Check sheet for the modelled part. Datum: model origin and axes. Units: mm. A direction names the side the tool comes from. Coordinates: 2 decimals unless noted, no trailing zeros. Write each loop counter-clockwise with the first axis right and the second up, starting at its lowest first coordinate (ties: lowest second). Pieces come first, ordered by that corner, then holes. Notation, with made-up numbers: M 11.25,77 L 60.25,77 A14 ccw 60.25,89 Z; hole C 11.5,52 d8. An arc over 180 degrees is marked long. Answer as CSV lines item,"result". Start each with the question number.
1) Section check A-A (z = -75). Record the cut outline in (x, y).
2) Access from +Z, -Z, +X, -X, +Y, -Y to the whole of each face (thin tool, end or side, straight path). Record for faces 1 (the flat face through (-27.477, 55, -64)), 2 (the flat face through (-28, 60, -53)).
3) Draft check along X on faces 3 (the flat face through (-37.477, 5, -64)), 4 (the cylindrical face through (4.78, 54.93, 1.5)), 5 (the flat face through (3.486, 29.58, -124.467)), 6 (the flat face through (-28, 0, -53)). Enter one of: +X half, -X half, draft (parallel to the pull), parting line (faces both ways), or undercut.
4) Section check B-B (x = 16). Record the cut outline in (y, z), and give its area (3 significant figures).
5) Material ranges on L1, parallel to Y at x = -31.5, z = -87; L2, parallel to X at y = 56, z = -61; L3, parallel to Z at x = 9, y = 3.5, recorded low to high. Write a range as [from, to].
6) Go/stop test with flat-tipped pins: pin 1 Ø12 at (y, z) = (48.5, -104) entering from +X; pin 2 Ø3 at (x, y) = (9.5, 17.5) entering from +Z; pin 3 Ø1 at (x, y) = (-7, 13) entering from -Z; pin 4 Ø5 at (y, z) = (10, -46) entering from +X. Record where each tip stops, or that it passes through.
7) Section check C-C (x = -5). Record the cut outline in (y, z), and give its area (3 significant figures).
8) Section check D-D (y = 6). Record the cut outline in (x, z).
from build123d import *

# Parameters (mm, degrees)
SKETCH_1_R          = 5
EXTRUDE_1_DEPTH     = 60
SKETCH_3_W          = 37.476659403
SKETCH_3_H          = 40
SKETCH_3_W_2        = 53
SKETCH_3_W_3        = 50.064849854
CUT_EXTRUDE_1_DEPTH = 58
EXTRUDE_2_DEPTH     = 40


with BuildPart() as part:
    # Sketch 1 → Extrude 1 (new body)
    with BuildSketch(Plane(origin=(0, 0, 0), x_dir=(1, 0, 0), z_dir=(0, 1, 0))):
        with BuildLine():
            Line((0, 0), (-37.476659403, 37.476659403))
            Line((-37.476659403, 37.476659403), (-37.476659403, 90.476659403))
            Line((-37.476659403, 90.476659403), (0, 127.953318806))
            Line((0, 127.953318806), (7.071067812, 120.882250994))
            Line((7.071067812, 120.882250994), (-27.476659403, 86.334523779))
            Line((-27.476659403, 86.334523779), (-27.476659403, 41.618795027))
            Line((-27.476659403, 41.618795027), (7.071067812, 7.071067812))
            ThreePointArc((7.071067812, 7.071067812), (16.730326075, -9.659258263), (0, 0))
        make_face()
        with Locations(Location((9.659258263, -2.588190451, 0), (0, 0, 270))):
            Circle(SKETCH_1_R, mode=Mode.SUBTRACT)
    extrude(amount=EXTRUDE_1_DEPTH)

    # Sketch 3 → Cut-Extrude 1 (cut)
    with BuildSketch(Plane.ZY.offset(37.476659403)):
        with Locations((-109.214989105, 30)):
            Rectangle(SKETCH_3_W, SKETCH_3_H)
        with Locations((-63.976659403, 30)):
            Rectangle(SKETCH_3_W_2, SKETCH_3_H)
        with Locations((-12.444234476, 30)):
            Rectangle(SKETCH_3_W_3, SKETCH_3_H)
    extrude(amount=-CUT_EXTRUDE_1_DEPTH, mode=Mode.SUBTRACT)


with BuildPart() as cut_extrude_1_piece_1:
    # of the separate pieces the step leaves, piece 1, a body of its own (cut_extrude_1_pieces)
    add(part.part.solids().sort_by_distance((7.071067812, 0, -7.071067812))[0])



with BuildPart() as cut_extrude_1_piece_2:
    # of the separate pieces the step leaves, piece 2, a body of its own (cut_extrude_1_pieces)
    add(part.part.solids().sort_by_distance((0, 50, 0))[0])


with BuildPart() as cut_extrude_1_piece_1_1:
    add(cut_extrude_1_piece_1.part)

    add(cut_extrude_1_piece_2.part)  # Extrude 2 merges Cut-Extrude 1 piece 2
    # Sketch 4 → Extrude 2 (add)
    with BuildSketch(Plane(origin=(0, 10, 0), x_dir=(1, 0, 0), z_dir=(0, 1, 0))):
        Polygon((0, 127.953318806), (7.071067812, 120.882250994), (0, 113.811183182), (-7.071067812, 120.882250994), align=None)
    extrude(amount=EXTRUDE_2_DEPTH)


solid = cut_extrude_1_piece_1_1.part
Results found:
1,outline,"M -37.48,0 L -27.48,0 L -27.48,10 L -37.48,10 Z; M -37.48,50 L -27.48,50 L -27.48,60 L -37.48,60 Z"
2,face 1,"+X, +Y, -Y"
2,face 2,"+Z, -Z, +X, -X, +Y"
3,face 3,"-X half"
3,face 4,"undercut"
3,face 5,"+X half"
3,face 6,"draft"
4,outline,"M 0,-5.14 L 10,-5.14 L 10,10.32 L 0,10.32 Z; M 50,-5.14 L 60,-5.14 L 60,10.32 L 50,10.32 Z"
4,area,"309 mm2"
5,L1,"y = [0, 10], [50, 60]"
5,L2,"x = [-37.48, -27.48]"
5,L3,"z = [-7.39, -2.37], [7.54, 12.57]"
6,pin 1,"stops at x = -4"
6,pin 2,"passes through"
6,pin 3,"stops at z = -121.45"
6,pin 4,"stops at x = -27.48"
7,outline,"M 0,-122.95 L 60,-122.95 L 60,-108.81 L 50,-108.81 L 50,-118.81 L 10,-118.81 L 10,-108.81 L 0,-108.81 Z; M 0,-19.14 L 10,-19.14 L 10,-5 L 0,-5 Z; M 50,-19.14 L 60,-19.14 L 60,-5 L 50,-5 Z"
7,area,"731 mm2"
8,outline,"M -37.48,-90.48 L 0,-127.95 L 7.07,-120.88 L -27.48,-86.33 L -27.48,-41.62 L 7.07,-7.07 A10 ccw long 0,0 L -37.48,-37.48 Z; hole C 9.66,2.59 d10"
